Autodesk Inventor part; units mm, degrees
ref_plane "YZ Plane" through (0, 0, 0) normal (1, 0, 0) x (0, 1, 0)
ref_plane "XZ Plane" through (0, 0, 0) normal (0, 1, 0) x (-1, 0, 0)
ref_plane "XY Plane" through (0, 0, 0) normal (0, 0, 1) x (1, 0, 0)
sketch "Boceto1" plane through (0, 0, 0) normal (0, 0, 1) x (1, 0, 0)
  circle A0 centre (0, 0) radius 24
  dimension "d0" = 48
extrude "Extrusión1" add sketch "Boceto1" against normal blind 250
shell "Vaciado1" thickness 2 removed faces 2 at (5.9881, 2.1306, 0) at (5.9881, 2.1306, -250)
sketch "Boceto2" plane through (0, 0, 0) normal (1, 0, 0) x (0, 1, 0)
  line L0 (-24, -250) -> (24, -250)
  line L1 (-24, 0) -> (24, 0)
  line L2 (-24, 0) -> (24, 0)
  line L3 (0, 0) -> (10, 0)
  line L4 (10, 0) -> (10, -50)
  line L5 (10, -50) -> (0, -50)
  line L6 (0, -50) -> (0, 0)
  line L7 (0, 0) -> (-10, 0)
  line L8 (-10, 0) -> (-10, -50)
  line L9 (-10, -50) -> (0, -50)
  line L10 (0, -50) -> (0, 0)
  dimension "d4" = 10
  dimension "d5" = 50
  dimension "d6" = 10
  dimension "d7" = 50
extrude "Extrusión2" cut sketch "Boceto2" along normal mid plane 60
properties part number "Cañón" material "Tuberías de PVC"
Geometry check sheet. Reference: the model listing, model coordinates, mm. A direction names the side the tool comes from. Coordinates: 2 decimals unless noted, no trailing zeros. Order: outer loops, then holes, each group sorted by start corner. A loop starts at its lowest first (then second) coordinate and runs counter-clockwise, first axis right, second up. Notation, with made-up numbers: (58, -12) - (98, -12) arc R30 ccw to (98, 23) - close; hole circle Ø9 at (38, 69.5). An arc over 180 degrees is marked (long way). Answer in a Markdown table with one row per item. Add a question column.
1) Set-up check for faces 1 (the flat face through (22.3, -0.1, -50)), 2 (the flat face through (-0.1, -22.2, 0)): record each of +Z, -Z, +X, -X, +Y, -Y from which the full face is reachable in a straight line by a thin tool's end or side.
2) Release check for a two-part mould opening along X. For faces 3 (the cylindrical face through (-23.977, 1.055, -123.25)), 4 (the flat face through (-0.1, 22.2, 0)), 5 (the cylindrical face through (-21.98, 0.97, -123.25)) record: +X half, -X half, draft (parallel to the pull), parting line (faces both ways), or undercut.
3) Gauge pin test, flat ends, axial feed: P1, Ø12, axis at x = -3, z = -142, coming from the +Y side; P2, Ø1.8, axis at x = -20.5, z = -29, coming from the -Y side; P3, Ø5, axis at x = 21, y = -4, coming from the +Z side. Record the tip position at first contact, or that the pin passes through.
4) Cross-section at A-A, the plane x = 0. Record the cut outline in (y, z), then the cut area to 3 significant figures.
5) Cross-section at C-C, the plane z = -190.5. Record the cut outline in (x, y), then the cut area to 3 significant figures.
6) Cross-section at B-B, the plane y = 0. Record the cut outline in (x, z), then the cut area to 3 significant figures.
7) Material ranges on line 1 along X through (y, z) = (0, -189.5); line 2 along X through (y, z) = (14, -64), recorded low to high. Write a range as [from, to].
Check result:
| question | item | result |
|---|---|---|
| 1 | face 1 | +Z, +X, -X |
| 1 | face 2 | +Z, +X, -X, +Y, -Y |
| 2 | face 3 | parting line |
| 2 | face 4 | draft |
| 2 | face 5 | undercut |
| 3 | P1 | stops at y = 24 |
| 3 | P2 | stops at y = -13.85 |
| 3 | P3 | stops at z = -50 |
| 4 | outline | (-24, -250) - (-22, -250) - (-22, 0) - (-24, 0) - close; (22, -250) - (24, -250) - (24, 0) - (22, 0) - close |
| 4 | area | 1,000 mm² |
| 5 | outline | circle Ø48 at (0, 0); hole circle Ø44 at (0, 0) |
| 5 | area | 289 mm² |
| 6 | outline | (-24, -250) - (-22, -250) - (-22, -50) - (-24, -50) - close; (22, -250) - (24, -250) - (24, -50) - (22, -50) - close |
| 6 | area | 800 mm² |
| 7 | line 1 | x = [-24, -22], [22, 24] |
| 7 | line 2 | x = [-19.49, -16.97], [16.97, 19.49] |
